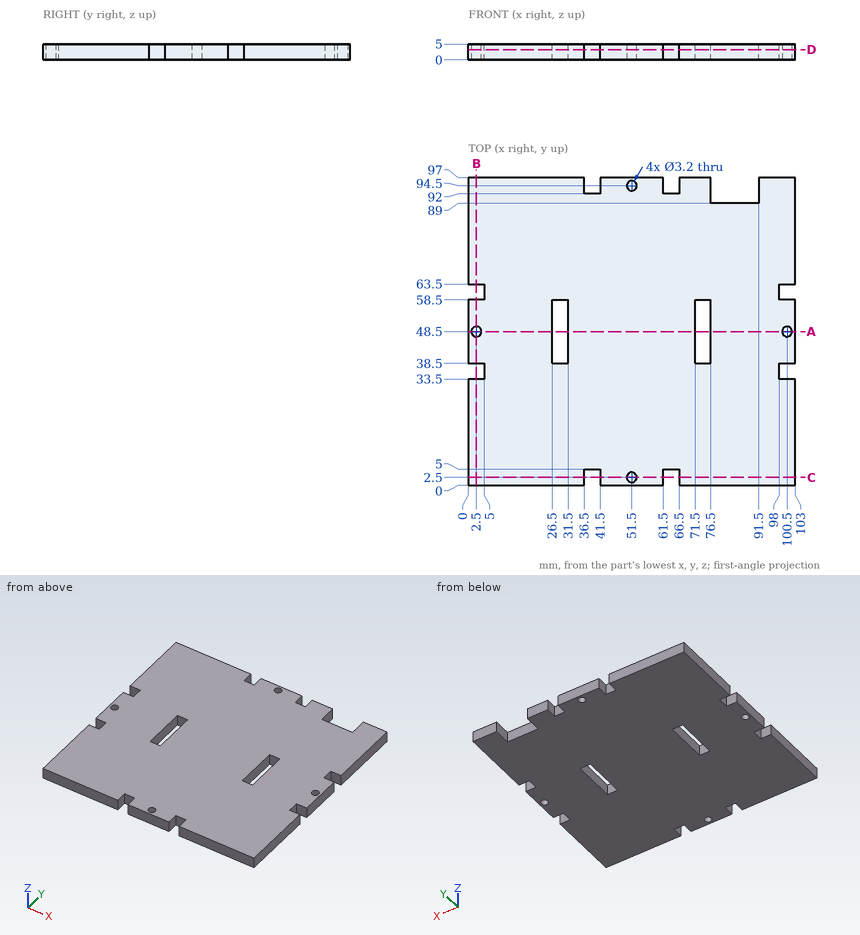
Design review of the part shown in the three views and the two pictorial views. Dimensions are in mm from the part's minimum x, y and z. Give positions to 0.01 mm unless a question says otherwise; leave off trailing zeros. Loops run counter-clockwise (first coordinate to the right, second up) from the corner with the lowest first, then second, coordinate; pieces in that order, holes last. Notation, with made-up numbers: (85, 39) - (103, 39) arc R16 cw to (103, 67) - close; hole circle Ø5 at (69, 3.25). An arc over 180 degrees is marked (long way). Answer as a JSON object with one key per item and string values.
Q1. Add section A-A on y = 48.5. State the section outline as (x, z) points, plus the area to 3 significant figures.
Worked out:
{"outline": "(0, 0) - (0.9, 0) - (0.9, 5) - (0, 5) - close; (4.1, 0) - (26.5, 0) - (26.5, 5) - (4.1, 5) - close; (31.5, 0) - (71.5, 0) - (71.5, 5) - (31.5, 5) - close; (76.5, 0) - (98.9, 0) - (98.9, 5) - (76.5, 5) - close; (102.1, 0) - (103, 0) - (103, 5) - (102.1, 5) - close", "area": "433 mm^2"}
Q2. Add section B-B on x = 2.5. State the section outline as (y, z) points.
Worked out:
{"outline": "(0, 0) - (33.5, 0) - (33.5, 5) - (0, 5) - close; (38.5, 0) - (46.9, 0) - (46.9, 5) - (38.5, 5) - close; (50.1, 0) - (58.5, 0) - (58.5, 5) - (50.1, 5) - close; (63.5, 0) - (97, 0) - (97, 5) - (63.5, 5) - close"}
Q3. To check wall thickness, follow line 1 along X through (y, z) = (55, 0.2); line 2 along X through (y, z) = (94.5, 1.2); line 3 along Y through (x, z) = (100.5, 2.35). State the ranges of each line that lie inside material, in increasing order.
Worked out:
{"line 1": "x = 0 to 26.5, 31.5 to 71.5, 76.5 to 103", "line 2": "x = 0 to 36.5, 41.5 to 49.9, 53.1 to 61.5, 66.5 to 76.5, 91.5 to 103", "line 3": "y = 0 to 33.5, 38.5 to 46.9, 50.1 to 58.5, 63.5 to 97"}
Q4. Add section D-D on z = 3.25. Count the separate pieces of the cut face and the enclosed holes in it, plus the area to 3 significant figures.
Worked out:
{"separate pieces": "1", "enclosed holes": "6", "area": "9,440 mm^2"}
Q5. Add section C-C on y = 2.5. State the section outline as (x, z) points.
Worked out:
{"outline": "(0, 0) - (36.5, 0) - (36.5, 5) - (0, 5) - close; (41.5, 0) - (49.9, 0) - (49.9, 5) - (41.5, 5) - close; (53.1, 0) - (61.5, 0) - (61.5, 5) - (53.1, 5) - close; (66.5, 0) - (103, 0) - (103, 5) - (66.5, 5) - close"}
Q6. Insertion check: pin 1 (1.5 mm diameter, centred on y = 60, z = 2, fed in from +X); pin 2 (1.5 mm diameter, centred on x = 90, z = 2.5, fed in from +Y). Each pin has a flat end and moves straight along its axis. Give the tip position at first contact, or say it passes through.
Worked out:
{"pin 1": "stops at x = 98", "pin 2": "stops at y = 89"}
